from build123d import *

# Parameters (mm, degrees)
SKETCH3_W           = 355.6
SKETCH3_H           = 177.8
BOSS_EXTRUDE1_DEPTH = 508
SKETCH4_R           = 31.75
CUT_EXTRUDE1_DEPTH  = 627.433212721
CHAMFER1_START      = -64
CHAMFER1_OUTLINE_W  = 75
CHAMFER1_OUTLINE_H  = 358
CHAMFER1_DEPTH      = 37.059231637
CHAMFER2_START      = -64
CHAMFER2_OUTLINE_W  = 75
CHAMFER2_OUTLINE_H  = 358
CHAMFER2_DEPTH      = 37.059231637
CHAMFER3_START      = 386.151013206
CHAMFER3_OUTLINE_W  = 75
CHAMFER3_OUTLINE_H  = 358
CHAMFER3_DEPTH      = 36.848986794
CHAMFER4_START      = 386.151013206
CHAMFER4_OUTLINE_W  = 75
CHAMFER4_OUTLINE_H  = 358
CHAMFER4_DEPTH      = 36.848986794
FILLET1_R           = 10
SKETCH5_R           = 76.2
CUT_EXTRUDE2_DEPTH  = 22.86
SKETCH7_W           = 342.323707946
SKETCH7_H           = 64.688657288
BOSS_EXTRUDE3_DEPTH = 177.8
SKETCH8_W           = 152.017430594
SKETCH8_H           = 316.368655432
CUT_EXTRUDE3_DEPTH  = 55.88
BOSS_EXTRUDE5_DEPTH = 55.88
SKETCH11_W          = 113.282529032
SKETCH11_H          = 39.308418544
BOSS_EXTRUDE6_DEPTH = 76.2
FILLET2_R           = 10.16
FILLET3_R           = 12.7
FILLET4_R           = 12.7
FILLET5_R           = 12.7
SKETCH12_R          = 24.948838793
BOSS_EXTRUDE7_DEPTH = 25.4
FILLET6_R           = 7.62
SKETCH13_R          = 12.609032653
BOSS_EXTRUDE8_DEPTH = 12.7
FILLET7_R           = 7.62


with BuildPart() as part:
    # Sketch3 → Boss-Extrude1 (new body)
    with BuildSketch(Plane(origin=(0, 0, 0), x_dir=(0, 0, -1), z_dir=(1, 0, 0))):
        Rectangle(SKETCH3_W, SKETCH3_H)
    extrude(amount=BOSS_EXTRUDE1_DEPTH)

    # Sketch4 → Cut-Extrude1 (cut, symmetric)
    with BuildSketch(Plane.XY.offset(177.8)):
        with Locations((101.6, 0)):
            Circle(SKETCH4_R)
    cut_extrude1 = extrude(amount=CUT_EXTRUDE1_DEPTH, both=True, mode=Mode.SUBTRACT)

    # Mirror1: Cut-Extrude1 across plane
    add(cut_extrude1.mirror(Plane.ZY.offset(-254)), mode=Mode.SUBTRACT)

    # Chamfer1: read off the stored shape, not the designer's step
    # Chamfer1 outline → Chamfer1 (cut)
    with BuildSketch(Plane(origin=(0, 0, 0), x_dir=(0.7071067811865471, 0.707106781186548, 0), z_dir=(0.707106781186548, -0.707106781186547, 0)).offset(CHAMFER1_START)):
        with Locations((62.5, 0)):
            Rectangle(CHAMFER1_OUTLINE_W, CHAMFER1_OUTLINE_H)
    extrude(amount=CHAMFER1_DEPTH, mode=Mode.SUBTRACT)

    # Chamfer2: read off the stored shape, not the designer's step
    # Chamfer2 outline → Chamfer2 (cut)
    with BuildSketch(Plane(origin=(0, 0, 0), x_dir=(0.707106781186548, -0.707106781186547, 0), z_dir=(0.707106781186547, 0.707106781186548, 0)).offset(CHAMFER2_START)):
        with Locations((62.5, 0)):
            Rectangle(CHAMFER2_OUTLINE_W, CHAMFER2_OUTLINE_H)
    extrude(amount=CHAMFER2_DEPTH, mode=Mode.SUBTRACT)

    # Chamfer3: read off the stored shape, not the designer's step
    # Chamfer3 outline → Chamfer3 (cut)
    with BuildSketch(Plane(origin=(0, 0, 0), x_dir=(0.707106781186548, -0.707106781186547, 0), z_dir=(0.707106781186547, 0.707106781186548, 0)).offset(CHAMFER3_START)):
        with Locations((296.5, 0)):
            Rectangle(CHAMFER3_OUTLINE_W, CHAMFER3_OUTLINE_H)
    extrude(amount=CHAMFER3_DEPTH, mode=Mode.SUBTRACT)

    # Chamfer4: read off the stored shape, not the designer's step
    # Chamfer4 outline → Chamfer4 (cut)
    with BuildSketch(Plane(origin=(0, 0, 0), x_dir=(0.707106781186548, 0.707106781186547, 0), z_dir=(0.707106781186547, -0.707106781186548, 0)).offset(CHAMFER4_START)):
        with Locations((296.5, 0)):
            Rectangle(CHAMFER4_OUTLINE_W, CHAMFER4_OUTLINE_H)
    extrude(amount=CHAMFER4_DEPTH, mode=Mode.SUBTRACT)

    # Fillet1
    fillet1_edges = [part.edges().sort_by_distance(p)[0] for p in [
        (50.8, 88.9, 0),
        (50.8, -88.9, 0),
        (254, 88.9, -177.8),
        (254, 88.9, 177.8),
        (457.2, 88.9, 0),
        (254, -88.9, 177.8),
        (254, -88.9, -177.8),
        (457.2, -88.9, 0),
    ]]
    fillet(fillet1_edges, radius=FILLET1_R)

    # Sketch5 → Cut-Extrude2 (cut)
    with BuildSketch(Plane(origin=(0, 88.9, 0), x_dir=(1, 0, 0), z_dir=(0, 1, 0))):
        with Locations(Location((254, 0, 0), (0, 0, 270))):
            Circle(SKETCH5_R)
    extrude(amount=-CUT_EXTRUDE2_DEPTH, mode=Mode.SUBTRACT)

    # Sketch7 → Boss-Extrude3 (add)
    with BuildSketch(Plane.ZY):
        Rectangle(SKETCH7_W, SKETCH7_H)
    extrude(amount=BOSS_EXTRUDE3_DEPTH)

    # Sketch8 → Cut-Extrude3 (cut)
    with BuildSketch(Plane(origin=(0, 32.344328644, 0), x_dir=(1, 0, 0), z_dir=(0, 1, 0))):
        with Locations((-88.9, 0)):
            Rectangle(SKETCH8_W, SKETCH8_H)
    extrude(amount=-CUT_EXTRUDE3_DEPTH, mode=Mode.SUBTRACT)

    # Sketch10 → Boss-Extrude5 (add)
    with BuildSketch(Plane.XY.offset(171.161853973)):
        Polygon((-177.8, -32.344328644), (40.8, -78.9), (20.4, -58.5), (-102.412744224, -32.344328644), align=None)
    boss_extrude5 = extrude(amount=-BOSS_EXTRUDE5_DEPTH)

    # Mirror2: Boss-Extrude5 across plane
    add(boss_extrude5.mirror(Plane.XY))

    # Sketch11 → Boss-Extrude6 (add)
    with BuildSketch(Plane(origin=(508, 0, 0), x_dir=(0, 0, -1), z_dir=(1, 0, 0))):
        Rectangle(SKETCH11_W, SKETCH11_H)
    extrude(amount=BOSS_EXTRUDE6_DEPTH)

    # Fillet2
    fillet2_edges = [part.edges().sort_by_distance(p)[0] for p in [
        (508, 0, -56.641264516),
        (546.1, -19.654209272, -56.641264516),
        (508, 19.654209272, 0),
        (546.1, 19.654209272, -56.641264516),
        (508, 0, 56.641264516),
        (546.1, 19.654209272, 56.641264516),
        (508, -19.654209272, 0),
        (546.1, -19.654209272, 56.641264516),
        (584.2, 0, -56.641264516),
        (584.2, 19.654209272, 0),
        (584.2, 0, 56.641264516),
        (584.2, -19.654209272, 0),
    ]]
    fillet(fillet2_edges, radius=FILLET2_R)

    # Fillet3
    fillet3_edges = [part.edges().sort_by_distance(p)[0] for p in [
        (508, 0, 177.8),
        (508, 38.1, 0),
        (508, 0, -177.8),
        (508, -38.1, 0),
    ]]
    fillet(fillet3_edges, radius=FILLET3_R)

    # Fillet4
    # the kernel refuses this fillet: 12.7 mm, written as the material it adds along each edge
    with BuildSketch(Plane(origin=(0, -32.344328644, 171.161853973), x_dir=(-1.269692375710673e-12, -1.0, 0), z_dir=(0, 0, -1))) as fillet4_piece_1:
        with BuildLine():
            CenterArc((12.7, 10.63326383), FILLET4_R, 180, 56.852413593)
            Line((0, 10.63326383), (-0.254, 10.63326383))
            Line((-0.254, 10.63326383), (-0.254, 0))
            Line((-0.254, 0), (0, -0.254))
            ThreePointArc((0, -0.254), (2.877835678, -0.254), (5.616784783, -0.212665277))
            Line((5.616784783, -0.212665277), (5.755671356, 0))
        make_face()
    extrude(amount=342.323707946)
    with BuildSketch(Plane(origin=(-12.891284703, -23.535671356, -158.184327716), x_dir=(0, 1, 0), z_dir=(0, 0, 1)), Plane(origin=(-164.908715297, -23.535671356, 158.184327716), x_dir=(0, 1, 0), z_dir=(0, 0, -1))) as fillet4_piece_2:
        with BuildLine():
            CenterArc((FILLET4_R, FILLET4_R), FILLET4_R, 180, 90)
            Line((0, FILLET4_R), (-FILLET4_R * 0.02, FILLET4_R))
            Line((-FILLET4_R * 0.02, FILLET4_R), (-FILLET4_R * 0.02, -FILLET4_R * 0.02))
            Line((-FILLET4_R * 0.02, -FILLET4_R * 0.02), (FILLET4_R, -FILLET4_R * 0.02))
            Line((FILLET4_R, -FILLET4_R * 0.02), (FILLET4_R, 0))
        make_face()
    extrude(amount=316.368655432)
    with BuildSketch(Plane(origin=(18.858715297, -23.535671356, 158.184327716), x_dir=(0, 1, 0), z_dir=(-1, 0, 0)), Plane(origin=(-164.908715297, -23.535671356, -158.184327716), x_dir=(0, 1, 0), z_dir=(1, 0, 0))) as fillet4_piece_3:
        with BuildLine():
            CenterArc((FILLET4_R, FILLET4_R), FILLET4_R, 180, 90)
            Line((0, FILLET4_R), (-FILLET4_R * 0.02, FILLET4_R))
            Line((-FILLET4_R * 0.02, FILLET4_R), (-FILLET4_R * 0.02, -FILLET4_R * 0.02))
            Line((-FILLET4_R * 0.02, -FILLET4_R * 0.02), (FILLET4_R, -FILLET4_R * 0.02))
            Line((FILLET4_R, -FILLET4_R * 0.02), (FILLET4_R, 0))
        make_face()
    extrude(amount=183.767430594)
    with BuildSketch(Plane(origin=(-164.908715297, -23.535671356, 189.934327716), x_dir=(0, 1, 0), z_dir=(0, 0, -1))) as fillet4_piece_4a_section:
        with BuildLine():
            CenterArc((FILLET4_R, FILLET4_R), FILLET4_R, 180, 90)
            Line((0, FILLET4_R), (-FILLET4_R * 0.02, FILLET4_R))
            Line((-FILLET4_R * 0.02, FILLET4_R), (-FILLET4_R * 0.02, -FILLET4_R * 0.02))
            Line((-FILLET4_R * 0.02, -FILLET4_R * 0.02), (FILLET4_R, -FILLET4_R * 0.02))
            Line((FILLET4_R, -FILLET4_R * 0.02), (FILLET4_R, 0))
        make_face()
    fillet4_piece_4a = extrude(amount=348.118655432, mode=Mode.PRIVATE)
    fillet4_piece_4a = split(fillet4_piece_4a, bisect_by=Plane(origin=(-164.908715297, -23.535671356, 158.184327716), z_dir=(0, 0, 1)), keep=Keep.TOP, mode=Mode.PRIVATE)
    with BuildSketch(Plane(origin=(-12.891284703, -23.535671356, 158.184327716), x_dir=(0, 1, 0), z_dir=(-1, 0, 0))) as fillet4_piece_4b_section:
        with BuildLine():
            CenterArc((FILLET4_R, FILLET4_R), FILLET4_R, 180, 90)
            Line((0, FILLET4_R), (-FILLET4_R * 0.02, FILLET4_R))
            Line((-FILLET4_R * 0.02, FILLET4_R), (-FILLET4_R * 0.02, -FILLET4_R * 0.02))
            Line((-FILLET4_R * 0.02, -FILLET4_R * 0.02), (FILLET4_R, -FILLET4_R * 0.02))
            Line((FILLET4_R, -FILLET4_R * 0.02), (FILLET4_R, 0))
        make_face()
    fillet4_piece_4b = extrude(amount=183.767430594, mode=Mode.PRIVATE)
    fillet4_piece_4b = split(fillet4_piece_4b, bisect_by=Plane(origin=(-164.908715297, -23.535671356, 158.184327716), z_dir=(-1, 0, 0)), keep=Keep.TOP, mode=Mode.PRIVATE)
    fillet4_piece_4 = fillet4_piece_4a & fillet4_piece_4b
    add(fillet4_piece_4)
    with BuildSketch(Plane(origin=(-164.908715297, -23.535671356, 158.184327716), x_dir=(0, 1, 0), z_dir=(0, 0, -1))) as fillet4_piece_5a_section:
        with BuildLine():
            CenterArc((FILLET4_R, FILLET4_R), FILLET4_R, 180, 90)
            Line((0, FILLET4_R), (-FILLET4_R * 0.02, FILLET4_R))
            Line((-FILLET4_R * 0.02, FILLET4_R), (-FILLET4_R * 0.02, -FILLET4_R * 0.02))
            Line((-FILLET4_R * 0.02, -FILLET4_R * 0.02), (FILLET4_R, -FILLET4_R * 0.02))
            Line((FILLET4_R, -FILLET4_R * 0.02), (FILLET4_R, 0))
        make_face()
    fillet4_piece_5a = extrude(amount=348.118655432, mode=Mode.PRIVATE)
    fillet4_piece_5a = split(fillet4_piece_5a, bisect_by=Plane(origin=(-164.908715297, -23.535671356, -158.184327716), z_dir=(0, 0, -1)), keep=Keep.TOP, mode=Mode.PRIVATE)
    with BuildSketch(Plane(origin=(-196.658715297, -23.535671356, -158.184327716), x_dir=(0, 1, 0), z_dir=(1, 0, 0))) as fillet4_piece_5b_section:
        with BuildLine():
            CenterArc((FILLET4_R, FILLET4_R), FILLET4_R, 180, 90)
            Line((0, FILLET4_R), (-FILLET4_R * 0.02, FILLET4_R))
            Line((-FILLET4_R * 0.02, FILLET4_R), (-FILLET4_R * 0.02, -FILLET4_R * 0.02))
            Line((-FILLET4_R * 0.02, -FILLET4_R * 0.02), (FILLET4_R, -FILLET4_R * 0.02))
            Line((FILLET4_R, -FILLET4_R * 0.02), (FILLET4_R, 0))
        make_face()
    fillet4_piece_5b = extrude(amount=183.767430594, mode=Mode.PRIVATE)
    fillet4_piece_5b = split(fillet4_piece_5b, bisect_by=Plane(origin=(-164.908715297, -23.535671356, -158.184327716), z_dir=(-1, 0, 0)), keep=Keep.TOP, mode=Mode.PRIVATE)
    fillet4_piece_5 = fillet4_piece_5a & fillet4_piece_5b
    add(fillet4_piece_5)

    # Fillet5
    fillet5_edges = [part.edges().sort_by_distance(p)[0] for p in [
        (-177.8, 32.344328644, 0),
    ]]
    fillet(fillet5_edges, radius=FILLET5_R)

    # Sketch12 → Boss-Extrude7 (add)
    with BuildSketch(Plane(origin=(0, 19.654209272, 0), x_dir=(1, 0, 0), z_dir=(0, 1, 0))):
        with Locations(Location((547.607631205, 0, 0), (0, 0, 90))):
            Circle(SKETCH12_R)
    extrude(amount=BOSS_EXTRUDE7_DEPTH)

    # Fillet6
    fillet6_edges = [part.edges().sort_by_distance(p)[0] for p in [
        (547.607631205, 45.054209272, 24.948838793),
    ]]
    fillet(fillet6_edges, radius=FILLET6_R)

    # Sketch13 → Boss-Extrude8 (add)
    with BuildSketch(Plane(origin=(0, 45.054209272, 0), x_dir=(1, 0, 0), z_dir=(0, 1, 0))):
        with Locations(Location((547.607631205, 0, 0), (0, 0, 270))):
            Circle(SKETCH13_R)
    extrude(amount=BOSS_EXTRUDE8_DEPTH)

    # Fillet7
    fillet7_edges = [part.edges().sort_by_distance(p)[0] for p in [
        (547.607631205, 57.754209272, -12.609032653),
    ]]
    fillet(fillet7_edges, radius=FILLET7_R)


solid = part.part
Source: CAD feature listing. Evaluate the final solid. Frame: model axes, mm. A direction names the side the tool comes from. Coordinates: 2 decimals unless noted, no trailing zeros. Loops run counter-clockwise (first coordinate to the right, second up) from the corner with the lowest first, then second, coordinate; pieces in that order, holes last. Notation, with made-up numbers: M -10.5,7.25 L 33.5,7.25 A19 cw 33.5,40.25 Z; hole C 19.25,44 d9. An arc over 180 degrees is marked long. Answer in a Markdown table with one row per item.
Q1. First-contact query: pin 1 (3 mm diameter, centred on y = 71, z = -51, fed in from +X); pin 2 (23.5 mm diameter, centred on x = -29.5, y = -52.5, fed in from +Z); pin 3 (10 mm diameter, centred on x = 458, z = 56.5, fed in from -Y); pin 4 (10.5 mm diameter, centred on x = 555, z = 1.5, fed in from +Y). Flat tips, straight axial feed; report the tip coordinate or a pass-through.
Answers below:
| item | result |
|---|---|
| pin 1 | stops at x = 476.6 |
| pin 2 | stops at z = 171.16 |
| pin 3 | stops at y = -88.9 |
| pin 4 | stops at y = 57.75 |
Q2. Ray query, probe 1 along Y at (x, z) = (406.4, -60); probe 2 along X at (y, z) = (-29, -140); probe 3 along X at (y, z) = (4, 144). Return the intervals inside material, ascending. Write a range as from..to.
Answers below:
| item | result |
|---|---|
| probe 1 | y = -88.9..-31.75, 31.75..88.9 |
| probe 2 | x = -177.8..88.67, 114.53..393.47, 419.33..508 |
| probe 3 | x = -177.8..-164.91, -12.89..70.1, 133.1..374.9, 437.9..508 |
Q3. Set-up query: faces 1 (the flat face through (-53, -50, -115.282)), 2 (the flat face through (-90, -23.536, -2)), 3 (the flat face through (-93, -32.344, -2)). Return all of +Z, -Z, +X, -X, +Y, -Y with unobstructed straight access to the full face (end or side cutting, diameter ignored); none if empty.
Answers below:
| item | result |
|---|---|
| face 1 | -X, -Y |
| face 2 | +Y |
| face 3 | none |
Q4. Section A-A on y = 0. State how many separate pieces and enclosed holes the cut face has, plus the area to 3 significant figures.
Answers below:
| item | result |
|---|---|
| separate pieces | 3 |
| enclosed holes | 1 |
| area | 157,000 mm^2 |
Q5. Section B-B on x = 101.6. Return the cut outline in (y, z), plus the area to 3 significant figures.
Answers below:
| item | result |
|---|---|
| outline | M -88.9,-167.8 A10 ccw -78.9,-177.8 L -31.75,-177.8 L -31.75,177.8 L -78.9,177.8 A10 ccw -88.9,167.8 Z; M 31.75,-177.8 L 78.9,-177.8 A10 ccw 88.9,-167.8 L 88.9,167.8 A10 ccw 78.9,177.8 L 31.75,177.8 Z |
| area | 40,600 mm^2 |
Q6. Draft query along X for faces 4 (the flat face through (-40.147, -45.605, -143.613)), 5 (the flat face through (560.4, 45.054, -1.2)), 6 (the flat face through (481.9, -64.2, 2.5)), 7 (the flat face through (-70.03, -55.296, 143.613)). Return one class per face: pulls with the +X half, pulls with the -X half, needs draft (parallel to the pull), parting line crosses it, or undercut.
Answers below:
| item | result |
|---|---|
| face 4 | undercut |
| face 5 | undercut |
| face 6 | pulls with the +X half |
| face 7 | pulls with the -X half |
